from build123d import *

# Parameters (mm, degrees)
EXTRUDE_1_DEPTH     = 24
SKETCH_2_R          = 1.6
CUT_EXTRUDE_1_DEPTH = 24
SKETCH_3_R          = 1.6
CUT_EXTRUDE_2_DEPTH = 24
FILLET_1_R          = 4


with BuildPart() as part:
    # 草图1 → 凸台-拉伸1 (new body)
    with BuildSketch(Plane.XY):
        Polygon((6, 112.691622655), (3, 112.691622655), (3, 101.691622655), (18, 101.691622655), (18, 104.691622655), (6, 104.691622655), align=None)
    extrude(amount=-EXTRUDE_1_DEPTH)

    # 草图2 → 切除-拉伸1 (cut)
    with BuildSketch(Plane(origin=(6, 0, 0), x_dir=(0, 0, -1), z_dir=(1, 0, 0))):
        with Locations(Location((6, 108.691622655, 0), (0, 0, 90))):
            Circle(SKETCH_2_R)
        with Locations(Location((18, 108.691622655, 0), (0, 0, 90))):
            Circle(SKETCH_2_R)
    extrude(amount=-CUT_EXTRUDE_1_DEPTH, mode=Mode.SUBTRACT)

    # 草图3 → 切除-拉伸2 (cut)
    with BuildSketch(Plane(origin=(0, 104.691622655, 0), x_dir=(1, 0, 0), z_dir=(0, 1, 0))):
        with Locations(Location((14, 6, 0), (0, 0, 180))):
            Circle(SKETCH_3_R)
        with Locations(Location((14, 18, 0), (0, 0, 180))):
            Circle(SKETCH_3_R)
    extrude(amount=-CUT_EXTRUDE_2_DEPTH, mode=Mode.SUBTRACT)

    # 圆角1
    fillet_1_edges = [part.edges().sort_by_distance(p)[0] for p in [
        (4.5, 112.691622655, -24),
        (4.5, 112.691622655, 0),
        (18, 103.191622655, -24),
        (18, 103.191622655, 0),
    ]]
    fillet(fillet_1_edges, radius=FILLET_1_R)


solid = part.part
Input: part model. Units: mm. Frame: model coordinates. A direction names the side the tool comes from. Round coordinates to 2 decimals unless told otherwise and drop trailing zeros. Loops run counter-clockwise (first coordinate to the right, second up) from the corner with the lowest first, then second, coordinate; pieces in that order, holes last. Notation, with made-up numbers: (-3.5, -20.5) -> (29.5, -20.5) arc R13 cw to (29.5, -3.5) -> close; hole circle Ø10 at (-12.5, 17.5). An arc over 180 degrees is marked (long way). Answer as a JSON object with one key per item and string values. Group by question number.
1) Ray query, L1, parallel to Z at x = 14, y = 102.65; L2, parallel to X at y = 106.25, z = -2; L3, parallel to Y at x = 16.5, z = -5. Return the intervals inside material, ascending.
2) Section query B-B on x = 5. Output: boundary loops of the cut face in (y, z).
3) Reachability of faces 1 (the flat face through (3, 107, -12)), 2 (the flat face through (6, 109, -12)) from +Z, -Z, +X, -X, +Y, -Y: full face, straight path, thin tool, end or side. Return the list, or none.
4) Pin query (flat end, axial travel): pin 1 (4 mm diameter, centred on y = 107, z = -18, fed in from +X); pin 2 (3.5 mm diameter, centred on x = 10, z = -7, fed in from +Y). Return the tip coordinate at first contact, or that it passes through.
5) Section query D-D on x = 13. Output: boundary loops of the cut face in (y, z), plus the area to 3 significant figures.
6) Section query C-C on y = 107.5. Output: boundary loops of the cut face in (x, z), plus the area to 3 significant figures.
7) Section query A-A on z = -6. Output: boundary loops of the cut face in (x, y).
8) Draft query along Y for faces 3 (the flat face through (12, 104.692, -12)), 4 (the cylindrical face through (4.52, 110.22, -17.52)), 5 (the flat face through (7, 104, 0)). Return one class per face: +Y half, -Y half, draft (parallel to the pull), parting line (faces both ways), or undercut.
Reply:
{
 "1": {"L1": "z = -24 to -19.6, -16.4 to -7.6, -4.4 to 0", "L2": "x = 3 to 6", "L3": "y = 101.69 to 104.69"},
 "2": {"outline": "(101.69, -24) -> (108.69, -24) arc R4 ccw to (112.69, -20) -> (112.69, -4) arc R4 ccw to (108.69, 0) -> (101.69, 0) -> close; hole circle Ø3.2 at (108.69, -18); hole circle Ø3.2 at (108.69, -6)"},
 "3": {"face 1": "+Z, -Z, -X, +Y, -Y", "face 2": "+Z, -Z, +X, +Y"},
 "4": {"pin 1": "stops at x = 6", "pin 2": "stops at y = 104.69"},
 "5": {"outline": "(101.69, -24) -> (104.69, -24) -> (104.69, -19.25) -> (101.69, -19.25) -> close; (101.69, -16.75) -> (104.69, -16.75) -> (104.69, -7.25) -> (101.69, -7.25) -> close; (101.69, -4.75) -> (104.69, -4.75) -> (104.69, 0) -> (101.69, 0) -> close", "area": "57.0 mm2"},
 "6": {"outline": "(3, -24) -> (6, -24) -> (6, -19.07) -> (3, -19.07) -> close; (3, -16.93) -> (6, -16.93) -> (6, -7.07) -> (3, -7.07) -> close; (3, -4.93) -> (6, -4.93) -> (6, 0) -> (3, 0) -> close", "area": "59.2 mm2"},
 "7": {"outline": "(3, 101.69) -> (12.4, 101.69) -> (12.4, 104.69) -> (6, 104.69) -> (6, 107.09) -> (3, 107.09) -> close; (3, 110.29) -> (6, 110.29) -> (6, 112.69) -> (3, 112.69) -> close; (15.6, 101.69) -> (18, 101.69) -> (18, 104.69) -> (15.6, 104.69) -> close"},
 "8": {"face 3": "+Y half", "face 4": "undercut", "face 5": "draft"}
}
